from build123d import *

# Parameters (mm, degrees)
SKETCH1_R           = 2.665
SKETCH1_R_2         = 1
BOSS_EXTRUDE1_DEPTH = 6.35


with BuildPart() as part:
    # Sketch1 → Boss-Extrude1 (new body)
    with BuildSketch(Plane.XY):
        with BuildLine():
            ThreePointArc((-12.7, 43.994090512), (-88.9, 0), (-12.7, -43.994090512))
            Line((-12.7, -43.994090512), (15.875, -27.49630657))
            ThreePointArc((15.875, -27.49630657), (31.75, 0), (15.875, 27.49630657))
            Line((15.875, 27.49630657), (-12.7, 43.994090512))
        make_face()
        with Locations((13.97, -24.196749782)):
            Circle(SKETCH1_R, mode=Mode.SUBTRACT)
        with Locations((13.97, 24.196749782)):
            Circle(SKETCH1_R, mode=Mode.SUBTRACT)
        with Locations((5.08, 0)):
            Circle(SKETCH1_R_2, mode=Mode.SUBTRACT)
        with Locations((10.16, 0)):
            Circle(SKETCH1_R_2, mode=Mode.SUBTRACT)
        Circle(SKETCH1_R_2, mode=Mode.SUBTRACT)
        with Locations((-27.94, 0)):
            Circle(SKETCH1_R, mode=Mode.SUBTRACT)
        with Locations((-10.16, 0)):
            Circle(SKETCH1_R_2, mode=Mode.SUBTRACT)
        with Locations((-5.08, 0)):
            Circle(SKETCH1_R_2, mode=Mode.SUBTRACT)
    extrude(amount=BOSS_EXTRUDE1_DEPTH)


solid = part.part
Can you work these out from the model? Positions are in its coordinate system, mm. Round coordinates to 2 decimals unless told otherwise and drop trailing zeros. Write each loop counter-clockwise with the first axis right and the second up, starting at its lowest first coordinate (ties: lowest second). Pieces come first, ordered by that corner, then holes. Notation, with made-up numbers: (82, 22) - (119, 22) arc R18 cw to (119, 34) - close; hole circle Ø5 at (27.25, -24). An arc over 180 degrees is marked (long way). Write each question's results on one line, items separated by ' | '. Start each with the question number.
1) Suppose I cut it at A-A (x = -27.94). List the corners of the cut face in (y, z) for me (3 decimals).
2) Suppose I cut it at D-D (y = -11.5). List the corners of the cut face in (x, z) for me, and give its area (3 significant figures).
3) Suppose I cut it at B-B (y = 25.5). List the corners of the cut face in (x, z) for me, and give its area (3 significant figures).
4) Suppose I cut it at C-C (z = 1). Give the number of separate pieces and of enclosed holes in the cut face, and give its area (3 significant figures).
5) We'd pull the mould along Y, two halves only. Please class faces 1 (the flat face through (1.39, -35.86, 3.13)), 2 (the cylindrical face through (31.747, -0.465, 3.131)), 3 (the cylindrical face through (11.308, -24.08, 3.131)): released by +Y, released by -Y, zero draft, split by the parting line, or undercut.
6) For pin 1 Ø3 at (x, z) = (-43.5, 4.5) entering from -Y; pin 2 Ø3 at (x, z) = (13.5, 3) entering from +Y; pin 3 Ø1 at (y, z) = (24.5, 5) entering from -X, each with a flat end and sliding along its axis, tell me the tip position at first contact or that it passes through.
7) Please list where these lines run through material, in increasing order: line 1 (Y direction, x = 12, z = 6); line 2 (Y direction, x = -27, z = 6); line 3 (Y direction, x = 9.5, z = 2).
Here are the results:
1) outline: (-49.774, 0) - (-2.665, 0) - (-2.665, 6.35) - (-49.774, 6.35) - close; (2.665, 0) - (49.774, 0) - (49.774, 6.35) - (2.665, 6.35) - close
2) outline: (-87.58, 0) - (29.59, 0) - (29.59, 6.35) - (-87.58, 6.35) - close | area: 744 mm2
3) outline: (-82.04, 0) - (11.65, 0) - (11.65, 6.35) - (-82.04, 6.35) - close; (16.29, 0) - (18.92, 0) - (18.92, 6.35) - (16.29, 6.35) - close | area: 612 mm2
4) separate pieces: 1 | enclosed holes: 8 | area: 9,100 mm2
5) face 1: released by -Y | face 2: split by the parting line | face 3: undercut
6) pin 1: stops at y = -50.65 | pin 2: stops at y = 29.73 | pin 3: stops at x = -82.87
7) line 1: y = -29.73 to -25.99, -22.4 to 22.4, 25.99 to 29.73 | line 2: y = -49.57 to -2.49, 2.49 to 49.57 | line 3: y = -31.18 to -0.75, 0.75 to 31.18
